Geometry: see drawing. Coordinates: mm, zero at the bounding-box minimum. A direction names the side the tool comes from. Round coordinates to 2 decimals unless told otherwise and drop trailing zeros. Loops run counter-clockwise (first coordinate to the right, second up) from the corner with the lowest first, then second, coordinate; pieces in that order, holes last.
(1) Cut plane B-B, the plane y = 3.85. Output: boundary loops of the cut face in (x, z).
(2) Access query for the marked faces 4, 5 and 6. Directions: +Z, -Z, +X, -X, +Y, -Y. A direction counts if a zero-diameter tool reaches every point of the face in a straight line with its end or side. Return the directions, or none.
(3) Cut plane A-A, the plane z = 3.75. Output: boundary loops of the cut face in (x, y).
(4) Cut plane C-C, the plane x = 4.75. Output: boundary loops of the cut face in (y, z).
(5) First-contact query: pin 1 Ø0.6 at (x, y) = (4, 4) entering from -Z. Flat tip, straight axial feed; report the tip coordinate or a pass-through.
(6) Line query: line 1 (Y direction, x = 3.85, z = 2.5); line 2 (Z direction, x = 3, y = 0.5); line 3 (X direction, y = 4, z = 3.5). Output: solid intervals per line, ascending.
(7) Draft query along X for the marked faces 1, 2 and 3. Return one class per face: released by +X, released by -X, zero draft, split by the parting line, or undercut.
(8) Cut plane D-D, the plane z = 7. Output: boundary loops of the cut face in (x, y), and give its area (3 significant figures).
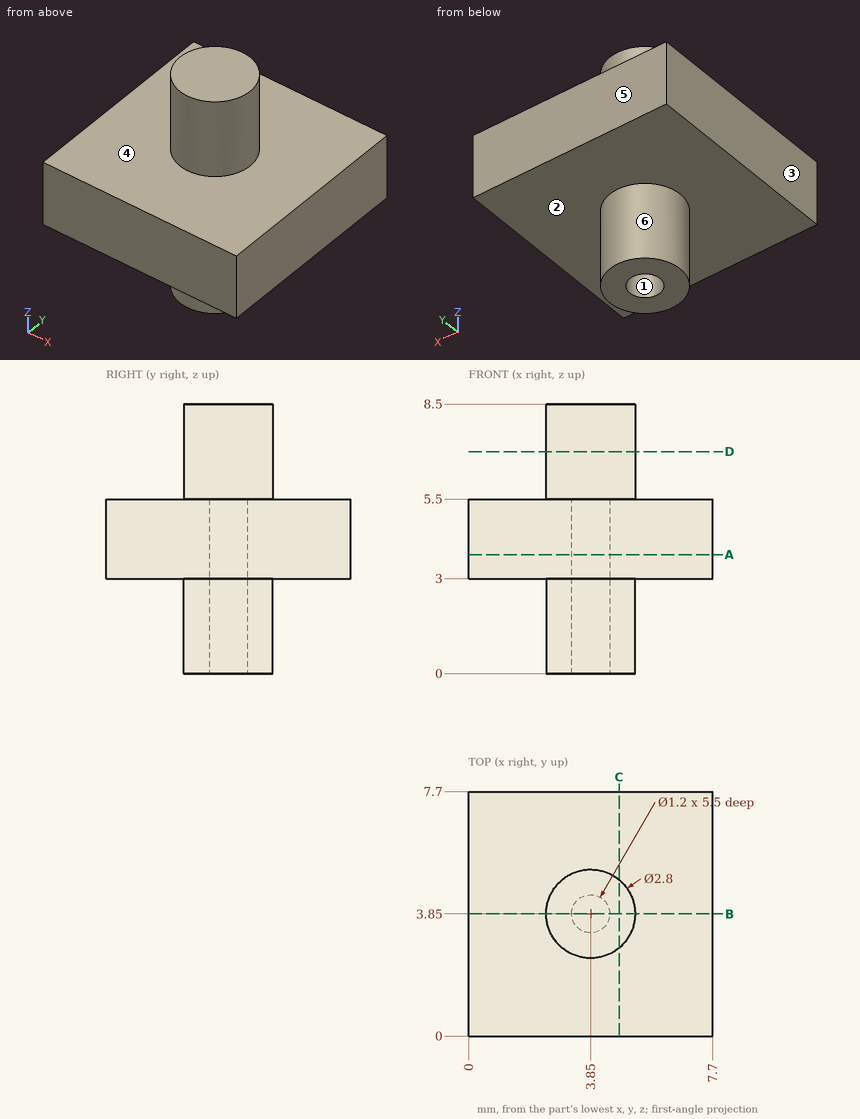
Reported:
1. outline: (0, 3) - (2.45, 3) - (2.45, 0) - (3.25, 0) - (3.25, 5.5) - (4.45, 5.5) - (4.45, 0) - (5.25, 0) - (5.25, 3) - (7.7, 3) - (7.7, 5.5) - (5.25, 5.5) - (5.25, 8.5) - (2.45, 8.5) - (2.45, 5.5) - (0, 5.5) - close
2. face 4: +Z
2. face 5: +Z, -Z, +X, -X, +Y
2. face 6: -Z
3. outline: (0, 0) - (7.7, 0) - (7.7, 7.7) - (0, 7.7) - close; hole circle Ø1.2 at (3.85, 3.85)
4. outline: (0, 3) - (2.78, 3) - (2.78, 0) - (4.92, 0) - (4.92, 3) - (7.7, 3) - (7.7, 5.5) - (4.92, 5.5) - (4.92, 8.5) - (2.78, 8.5) - (2.78, 5.5) - (0, 5.5) - close
5. pin 1: stops at z = 5.5
6. line 1: y = 2.45 to 3.25, 4.45 to 5.25
6. line 2: z = 3 to 5.5
6. line 3: x = 0 to 3.27, 4.43 to 7.7
7. face 1: undercut
7. face 2: zero draft
7. face 3: released by -X
8. outline: circle Ø2.8 at (3.85, 3.85)
8. area: 6.16 mm2
